For this review, take the finished solid that the model builds, in its own axes (mm). A direction names the side the tool comes from. Round coordinates to 2 decimals unless told otherwise and drop trailing zeros. Write each loop counter-clockwise with the first axis right and the second up, starting at its lowest first coordinate (ties: lowest second). Pieces come first, ordered by that corner, then holes. Notation, with made-up numbers: M -20,12 L 10,12 A32 cw 10,42 Z; hole C -8.5,57 d9. An arc over 180 degrees is marked long. Answer in a Markdown table with one row per item.
```python
from build123d import *

# Parameters (mm, degrees)
F0_R        = 5
F1_DEPTH    = 2
F2_R        = 8
F2_R_2      = 5
F3_DEPTH    = 8
F4_R        = 5
F4_R_2      = 4.1
F5_DEPTH    = 4
F6_S5_R     = 5
F6_T6_DEPTH = 9


# Not quite as in the source:
# - a fillet or chamfer that OpenCascade refuses, or shapes differently, is made with other operations: its cross-section is extruded or revolved along the edge and cut away or added


with BuildPart() as f1:
    # F0 (on Front) → F1 (new body)
    with BuildSketch(Plane.XZ):
        with BuildLine():
            ThreePointArc((-3.1857954632, -16.6988235294), (0, -13.8), (3.1857954632, -16.6988235294))
            ThreePointArc((3.1857954632, -16.6988235294), (0, 17), (-3.1857954632, -16.6988235294))
        make_face()
        Circle(F0_R, mode=Mode.SUBTRACT)
    extrude(amount=F1_DEPTH)

    # F2 (on Front) → F3 (join)
    with BuildSketch(Plane.XZ):
        Circle(F2_R)
        Circle(F2_R_2, mode=Mode.SUBTRACT)
    extrude(amount=F3_DEPTH)

    # F4 (on face) → F5 (join)
    with BuildSketch(Plane.XZ.offset(8)):
        Circle(F4_R)
        Circle(F4_R_2, mode=Mode.SUBTRACT)
    extrude(amount=-F5_DEPTH)

    # F6: chamfer of 1 on 1 edges, made by hand


with BuildPart() as f6_tool2:
    # F6_s3 → F6_t4 (revolve)
    with BuildSketch(Plane.XY):
        Polygon((5.1, -4), (4.1, -5), (4.1, -4), align=None)
    revolve(axis=Axis((0, -4, 0), (0, -1, 0)))

    # F6_s5 → F6_t6 (intersect, symmetric)
    with BuildSketch(Plane.XZ.offset(4.5)):
        Circle(F6_S5_R)
    extrude(amount=F6_T6_DEPTH, both=True, mode=Mode.INTERSECT)


with BuildPart() as f1_1:
    add(f1.part)

    # F6_t1: cut F6_tool2
    add(f6_tool2.part, mode=Mode.SUBTRACT)


solid = f1_1.part
```
Q1. Take a section at B-B (z = 0). State the section outline as (x, y) points, then the cut area to 3 significant figures.
Found:
| item | result |
|---|---|
| outline | M -17,-2 L -8,-2 L -8,-8 L -4.1,-8 L -4.1,-5 L -5,-4.1 L -5,0 L -17,0 Z; M 4.1,-8 L 8,-8 L 8,-2 L 17,-2 L 17,0 L 5,0 L 5,-4.1 L 4.1,-5 Z |
| area | 90.2 mm² |
Q2. Mouldability with a two-part tool opening along X and no side actions: class faces 1 (the face through (-0.1, -1, -13.8)), 2 (the face through (-1.73, -4.96, -7.81)), 3 (the face through (-4, -8, 2)) as +X half, -X half, draft (parallel to the pull), parting line (faces both ways), or undercut.
Found:
| item | result |
|---|---|
| face 1 | undercut |
| face 2 | parting line |
| face 3 | draft |
Q3. Take a section at D-D (x = 6.5). State the section outline as (y, z) points, then the cut area to 3 significant figures.
Found:
| item | result |
|---|---|
| outline | M -8,-4.66 L -2,-4.66 L -2,-15.71 L 0,-15.71 L 0,15.71 L -2,15.71 L -2,4.66 L -8,4.66 Z |
| area | 119 mm² |
Q4. Take a section at A-A (x = 0). State the section outline as (y, z) points.
Found:
| item | result |
|---|---|
| outline | M -8,-8 L -2,-8 L -2,-13.8 L 0,-13.8 L 0,-5 L -4.1,-5 L -5,-4.1 L -8,-4.1 Z; M -8,4.1 L -5,4.1 L -4.1,5 L 0,5 L 0,17 L -2,17 L -2,8 L -8,8 Z |
Q5. Insertion check: P1, Ø3, axis at x = 6, z = -4, coming from the +Y side; P2, Ø1.5, axis at x = -4, y = -3.5, coming from the +Z side; P3, Ø1.5, axis at x = -2, z = -13.5, coming from the -Y side; P4, Ø2, axis at x = -3, y = -7, coming from the +Z side. Each pin has a flat end and moves straight along its axis. Give the tip position at first contact, or say it passes through.
Found:
| item | result |
|---|---|
| P1 | y = 0 |
| P2 | z = 7.31 |
| P3 | y = -2 |
| P4 | z = 7.75 |
Q6. For probe 1 along Z at (x, y) = (0, -6.1); probe 2 along Z at (x, y) = (0, -3.95); probe 3 along Y at (x, z) = (-14, -5), list the stretches that pass through material, from the lowest coordinate up.
Found:
| item | result |
|---|---|
| probe 1 | -8 to -4.1, 4.1 to 8 |
| probe 2 | -8 to -5, 5 to 8 |
| probe 3 | -2 to 0 |
Q7. Take a section at C-C (y = -4.5). State the section outline as (x, z) points.
Found:
| item | result |
|---|---|
| outline | C 0,0 d16; hole C 0,0 d9.2 |
Q8. Machinability: for faces 4 (the face through (0.703, -0.986, 16.985)), 5 (the face through (-4.02, -2, -7.1)), which of the approach directions +Z, -Z, +X, -X, +Y, -Y give a long, thin tool a straight path to every point of the face, cutting with its end or side? Answer none if there is none.
Found:
| item | result |
|---|---|
| face 4 | +Y, -Y |
| face 5 | -Y |
